Verification items for the finished model (mm, model axes). A direction names the side the tool comes from. Round coordinates to 2 decimals unless told otherwise and drop trailing zeros. Write each loop counter-clockwise with the first axis right and the second up, starting at its lowest first coordinate (ties: lowest second). Pieces come first, ordered by that corner, then holes. Notation, with made-up numbers: M 55.5,10 L 91.5,10 A24 ccw 91.5,32 Z; hole C 57,-14.75 d8. An arc over 180 degrees is marked long. One line per item, written item: value. Start each with the question number.
Item 1: Section check C-C, the plane y = 37.5. Record the cut outline in (x, z).
Item 2: Tool access check on faces 1 (the face through (-20.9, 30.8, -4.6)), 2 (the face through (4, 41, 0)), 3 (the face through (4, 28.9, 0)). Record the directions out of +Z, -Z, +X, -X, +Y, -Y that give a thin tool (end or side, any length) a straight path to the whole face; none if there is none.
Item 3: Draft check along Z on faces 4 (the face through (0, 44.1, -4)), 5 (the face through (-9.911, 42.454, 0.176)), 6 (the face through (-20.9, 14.2, -4.6)). Enter one of: +Z half, -Z half, draft (parallel to the pull), parting line (faces both ways), or undercut.
Item 4: Thickness scan on probe 1 along X at (y, z) = (31.2, 0); probe 2 along Y at (x, z) = (6, -11.5); probe 3 along X at (y, z) = (7.5, 1). Record the ranges inside material, lowest first. Write a range as from..to.
Item 5: Gauge pin test, flat ends, axial feed: pin 1 (5 mm diameter, centred on x = 16, z = -14.5, fed in from +Y); pin 2 (6 mm diameter, centred on y = 15.5, z = 10.5, fed in from -X); pin 3 (10 mm diameter, centred on x = 0, z = 3.5, fed in from -Y); pin 4 (6 mm diameter, centred on x = 7.5, y = 24, fed in from +Z). Record the tip position at first contact, or that the pin passes through.
Item 6: Section check B-B, the plane y = 19. Record the cut outline in (x, z).
Item 7: Section check A-A, the plane z = 0. State how many separate pieces and enclosed holes the cut face has, then the cut area to 3 significant figures.
from build123d import *

# Parameters (mm, degrees)
SKETCH_1_R                = 21.4
SKETCH_1_R_2              = 18
EXTRUDE_1_DEPTH           = 32
SKETCH_13_R               = 2.5
CUT_EXTRUDE_1_DEPTH       = 54.544415829
HOLE_WIZARD_1_D           = 2.7
HOLE_WIZARD_1_CSINK_D     = 3
HOLE_WIZARD_1_CSINK_ANGLE = 90


with BuildPart() as part:
    # 草图1 → 凸台-拉伸1 (new body)
    with BuildSketch(Plane(origin=(0, 0, 0), x_dir=(1, 0, 0), z_dir=(0, 1, 0))):
        with Locations(Location((0, 0, 0), (0, 0, 270))):
            Circle(SKETCH_1_R)
        with Locations(Location((0, 0, 0), (0, 0, 270))):
            Circle(SKETCH_1_R_2, mode=Mode.SUBTRACT)
    extrude(amount=EXTRUDE_1_DEPTH)

    # 草图11 → 旋转-薄壁4 (revolve)
    with BuildSketch(Plane(origin=(0, 0, 0), x_dir=(0, 0, -1), z_dir=(1, 0, 0)), mode=Mode.PRIVATE) as revolve_4_sk:
        Polygon((0, 41), (-17, 41), (-18.006981843, 32), (0, 32), (0, 28.9), (-21.473174735, 28.9), (-19.772494289, 44.1), (0, 44.1), align=None)
    revolve(revolve_4_sk.sketch.rotate(Axis((0, 0, 0), (0, 1, 0)), 180), axis=Axis((0, 0, 0), (0, 1, 0)))

    # 草图13 → 切除-拉伸1 (cut, through all)
    with BuildSketch(Plane(origin=(0, 44.1, 0), x_dir=(1, 0, 0), z_dir=(0, 1, 0))):
        with Locations(Location((0, 0, 0), (0, 0, 270))):
            Circle(SKETCH_13_R)
    extrude(amount=-CUT_EXTRUDE_1_DEPTH, mode=Mode.SUBTRACT)

    # 打孔尺寸(%根据)内六角花形半沉头螺钉的类型1 (through all)
    with Locations(Plane(origin=(0, 44.1, -11.25), x_dir=(0, 0, 1), z_dir=(0, 1, 0))):
        with Locations((0, 0), (11.25, 11.25), (22.5, 0), (11.25, -11.25)):
            CounterSinkHole(HOLE_WIZARD_1_D / 2, HOLE_WIZARD_1_CSINK_D / 2, counter_sink_angle=HOLE_WIZARD_1_CSINK_ANGLE)


solid = part.part
Response values:
1. outline: C 0,0 d41.02; hole C 0,0 d34.78
2. face 1: +Y
2. face 2: none
2. face 3: -Y
3. face 4: draft
3. face 5: undercut
3. face 6: parting line
4. probe 1: x = -21.4..-12.6, -9.9..-2.5, 2.5..9.9, 12.6..21.4
4. probe 2: y = 28.9..32, 41..44.1
4. probe 3: x = -21.38..-17.97, 17.97..21.38
5. pin 1: stops at y = 44.1
5. pin 2: stops at x = -20.04
5. pin 3: stops at y = 28.9
5. pin 4: stops at z = 20.92
6. outline: C 0,0 d42.8; hole C 0,0 d36
7. separate pieces: 6
7. enclosed holes: 0
7. area: 445 mm2
